Input: part model. Units: mm. Frame: model coordinates. Face numbers are marked on the shaded views. A direction names the side the tool comes from. Give positions to 0.01 mm unless a question says otherwise; leave off trailing zeros. Loops run counter-clockwise (first coordinate to the right, second up) from the corner with the lowest first, then second, coordinate; pieces in that order, holes last.
from build123d import *

# Parameters (mm, degrees)
BOSS_EXTRUDE1_DEPTH = 26.8
SKETCH2_W           = 21.5
SKETCH2_H           = 43.5
SKETCH2_W_2         = 43.5
SKETCH2_H_2         = 21.5
CUT_EXTRUDE1_DEPTH  = 157.194070808
SKETCH3_R           = 1.15
BOSS_EXTRUDE2_DEPTH = 26.8
SKETCH3_2_R         = 1.15
CUT_EXTRUDE2_DEPTH  = 157.194070808
SKETCH4_R           = 1.15
CUT_EXTRUDE3_DEPTH  = 157.194070808
FILLET1_R           = 2.3
SKETCH6_R           = 1.75
CUT_EXTRUDE4_DEPTH  = 157.194070808
SKETCH7_R           = 3
CUT_EXTRUDE5_DEPTH  = 5


with BuildPart() as part:
    # Sketch1 → Boss-Extrude1 (new body)
    with BuildSketch(Plane.XY):
        Polygon((86.954468728, 12.865007186), (116.954468728, 12.865007186), (116.954468728, 100), (86.954468728, 100), (86.954468728, 42.865007186), (6.954468728, 42.865007186), (6.954468728, 100), (-23.045531272, 100), (-23.045531272, 12.865007186), (6.954468728, 12.865007186), align=None)
    extrude(amount=BOSS_EXTRUDE1_DEPTH)

    # Sketch2 → Cut-Extrude1 (cut, through all)
    with BuildSketch(Plane.XY.offset(26.8)):
        with Locations((-8.045531272, 41.615007186)):
            Rectangle(SKETCH2_W, SKETCH2_H)
        with Locations((73.204468728, 28.145492547)):
            Rectangle(SKETCH2_W_2, SKETCH2_H_2)
    extrude(amount=-CUT_EXTRUDE1_DEPTH, mode=Mode.SUBTRACT)

    # Sketch3 → Boss-Extrude2 (add, through all)
    with BuildSketch(Plane.XY.offset(26.8)):
        with Locations((-13.045531272, 14.565007186)):
            Circle(SKETCH3_R)
        with Locations((-3.045531272, 14.565007186)):
            Circle(SKETCH3_R)
        with Locations((-13.045531272, 65.665007186)):
            Circle(SKETCH3_R)
        with Locations((-3.045531272, 65.665007186)):
            Circle(SKETCH3_R)
    extrude(amount=-BOSS_EXTRUDE2_DEPTH)

    # Sketch3<2> → Cut-Extrude2 (cut, through all)
    with BuildSketch(Plane.XY.offset(26.8)):
        with Locations((-13.045531272, 14.565007186)):
            Circle(SKETCH3_2_R)
        with Locations((-3.045531272, 14.565007186)):
            Circle(SKETCH3_2_R)
        with Locations((-13.045531272, 65.665007186)):
            Circle(SKETCH3_2_R)
        with Locations(Location((-3.045531272, 65.665007186, 0), (0, 0, 180))):
            Circle(SKETCH3_2_R)
    extrude(amount=-CUT_EXTRUDE2_DEPTH, mode=Mode.SUBTRACT)

    # Sketch4 → Cut-Extrude3 (cut, through all)
    with BuildSketch(Plane.XY.offset(26.8)):
        with Locations((100.254468728, 23.145492547)):
            Circle(SKETCH4_R)
        with Locations(Location((100.254468728, 33.145492547, 0), (0, 0, 180))):
            Circle(SKETCH4_R)
        with Locations((49.154468728, 23.145492547)):
            Circle(SKETCH4_R)
        with Locations(Location((49.154468728, 33.145492547, 0), (0, 0, 180))):
            Circle(SKETCH4_R)
    extrude(amount=-CUT_EXTRUDE3_DEPTH, mode=Mode.SUBTRACT)

    # Fillet1
    fillet1_edges = [part.edges().sort_by_distance(p)[0] for p in [
        (6.954468728, 100, 13.4),
        (86.954468728, 100, 13.4),
        (116.954468728, 100, 13.4),
        (116.954468728, 12.865007186, 13.4),
        (-23.045531272, 12.865007186, 13.4),
        (-23.045531272, 100, 13.4),
        (116.954468728, 56.432503593, 26.8),
        (101.954468728, 100, 26.8),
        (86.954468728, 71.432503593, 26.8),
        (46.954468728, 42.865007186, 26.8),
        (6.954468728, 71.432503593, 26.8),
        (-8.045531272, 100, 26.8),
        (-23.045531272, 56.432503593, 26.8),
    ]]
    fillet(fillet1_edges, radius=FILLET1_R)

    # Sketch6 → Cut-Extrude4 (cut, through all)
    with BuildSketch(Plane.XY):
        with Locations((101.954468728, 90)):
            Circle(SKETCH6_R)
        with Locations((-8.045531272, 85)):
            Circle(SKETCH6_R)
        with Locations((26.954468728, 27.865007186)):
            Circle(SKETCH6_R)
    extrude(amount=CUT_EXTRUDE4_DEPTH, mode=Mode.SUBTRACT)

    # Sketch7 → Cut-Extrude5 (cut)
    with BuildSketch(Plane.XY.offset(26.8)):
        with Locations((-8.045531272, 85)):
            Circle(SKETCH7_R)
        with Locations((26.954468728, 27.865007186)):
            Circle(SKETCH7_R)
        with Locations((101.954468728, 90)):
            Circle(SKETCH7_R)
    extrude(amount=-CUT_EXTRUDE5_DEPTH, mode=Mode.SUBTRACT)


solid = part.part
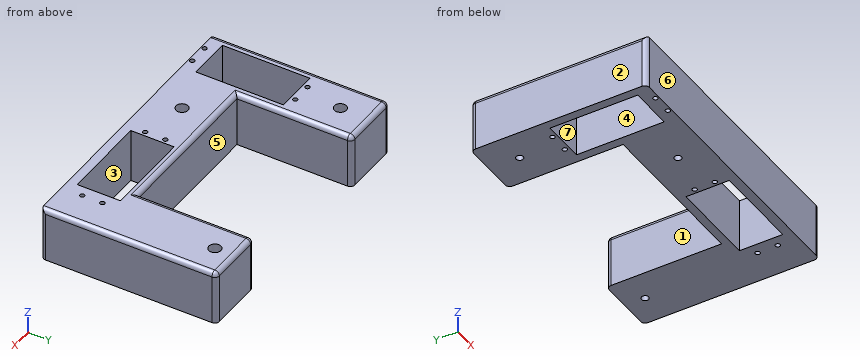
(1) Cut plane A-A (y = 68.5). Return the cut outline in (x, z), and give its area (3 significant figures).
Values follow:
outline: (-23.05, 0) - (6.95, 0) - (6.95, 24.5) arc R2.3 ccw to (4.65, 26.8) - (-20.75, 26.8) arc R2.3 ccw to (-23.05, 24.5) - close; (86.95, 0) - (116.95, 0) - (116.95, 24.5) arc R2.3 ccw to (114.65, 26.8) - (89.25, 26.8) arc R2.3 ccw to (86.95, 24.5) - close
area: 1,600 mm2
(2) Cut plane B-B (x = 66). Return the cut outline in (y, z) (1 decimal).
Values follow:
outline: (12.9, 0) - (17.4, 0) - (17.4, 26.8) - (12.9, 26.8) - close; (38.9, 0) - (42.9, 0) - (42.9, 24.5) arc R2.3 ccw to (40.6, 26.8) - (38.9, 26.8) - close
(3) Ray query, probe 1 along X at (y, z) = (30, 2.5); probe 2 along X at (y, z) = (85, 2.25); probe 3 along X at (y, z) = (42.5, 18.25). Return the intervals inside material, ascending.
Values follow:
probe 1: x = -23.05 to -18.8, 2.7 to 51.45, 94.95 to 116.95
probe 2: x = -23.05 to -9.8, -6.3 to 6.95, 86.95 to 116.95
probe 3: x = -23.05 to -18.8, 2.7 to 116.95
(4) Cut plane C-C (y = 36). Return the cut outline in (x, z), and give its area (3 significant figures).
Values follow:
outline: (-23.05, 0) - (-18.8, 0) - (-18.8, 26.8) - (-20.75, 26.8) arc R2.3 ccw to (-23.05, 24.5) - close; (2.7, 0) - (51.45, 0) - (51.45, 26.8) - (2.7, 26.8) - close; (94.95, 0) - (116.95, 0) - (116.95, 24.5) arc R2.3 ccw to (114.65, 26.8) - (94.95, 26.8) - close
area: 2,010 mm2
(5) Cut plane D-D (z = 2.5). Count the separate pieces of the cut face and the enclosed holes in it, and give its area (3 significant figures).
Values follow:
separate pieces: 1
enclosed holes: 13
area: 5,690 mm2
(6) Mould query, pull axis Y, two halves, no side actions, for the marked faces 4, 5, 6 and 7. Classes: +Y half, -Y half, draft (parallel to the pull), parting line (faces both ways), or undercut.
Values follow:
face 4: undercut
face 5: +Y half
face 6: -Y half
face 7: undercut
(7) Reachability of the marked faces 1, 2 and 3 from +Z, -Z, +X, -X, +Y, -Y: full face, straight path, thin tool, end or side. Return the list, or none.
Values follow:
face 1: +Z, -Z, +Y
face 2: +Z, -Z, -X, +Y, -Y
face 3: +Z, -Z
(8) Pin query (flat end, axial travel): pin 1 Ø13.5 at (x, z) = (64.5, 17) entering from +Y (3 decimals); pin 2 Ø1.8 at (x, y) = (-8.5, 84) entering from +Z. Return the tip coordinate at first contact, or that it passes through.
Values follow:
pin 1: stops at y = 42.865
pin 2: stops at z = 21.8
